```python
from build123d import *

# Parameters (mm, degrees)
SKETCH_R     = 11.1125
SKETCH003_R  = 11.1125
PAD_DEPTH    = 137
SKETCH004_W  = 152.4
SKETCH004_H  = 270.212156
PAD001_DEPTH = 0.508


with BuildPart() as part:
    # AdditivePipe: sweep along a path in Sketch001
    with BuildLine(Plane.YZ) as additivepipe_path:
        Line((0, 0), (279.4, 0))
        ThreePointArc((279.4, 0), (297.360512, -7.439488), (304.8, -25.4))
        Line((304.8, -25.4), (304.8, -254))
        ThreePointArc((304.8, -254), (297.360512, -271.960512), (279.4, -279.4))
        Line((279.4, -279.4), (184.15, -279.4))
        Line((184.15, -279.4), (184.15, -406.4))
        ThreePointArc((184.15, -406.4), (176.710512, -424.360512), (158.75, -431.8))
        Line((158.75, -431.8), (0, -431.8))
    # Sketch → AdditivePipe (sweep)
    with BuildSketch(Plane.XZ):
        Circle(SKETCH_R)
    sweep(path=additivepipe_path.line, transition=Transition.RIGHT)

    # Sketch003 (on DatumPlane) → Pad (new body)
    with BuildSketch(Plane(origin=(0, 69.85, -279.4), x_dir=(-1, 0, 0), z_dir=(0, 1, 0))):
        Circle(SKETCH003_R)
    extrude(amount=PAD_DEPTH)

    # Sketch004 → Pad001 (join, symmetric)
    with BuildSketch(Plane.YZ):
        with Locations((146.05, -138.737672)):
            Rectangle(SKETCH004_W, SKETCH004_H)
    extrude(amount=PAD001_DEPTH, both=True)


solid = part.part
```
CAD build for the part. Positions are in the model's coordinates, mm. A direction names the side the tool comes from. Give positions to 0.01 mm unless a question says otherwise; leave off trailing zeros. Put each result on its own line as item: value.
Q1. Tool access for faces 3 (the face through (-0.508, 145, -138)), 4 (the face through (-11.1, 183.66, -343.79)), 5 (the face through (0, 69.85, -233)), 6 (the face through (0.508, 145, -138)): list every direction of +Z, -Z, +X, -X, +Y, -Y with a clear straight run to the whole face (end or side of a thin tool).
Filled in:
face 3: -X, -Y
face 4: none
face 5: +X, -X, -Y
face 6: +X, -Y
Q2. Flat gauge pins, fed straight in: pin 1 (3 mm diameter, centred on x = -2, y = 67.5, fed in from +Z); pin 2 (4 mm diameter, centred on x = 1, z = -113, fed in from -Y); pin 3 (2 mm diameter, centred on y = 127.5, z = -71, fed in from -X). Where does each tip first touch, or does it go through?
Filled in:
pin 1: stops at z = 11.1
pin 2: stops at y = 69.85
pin 3: stops at x = -0.51
Q3. Mould opens along Z. For faces 1 (the face through (0, 0, -432)), 2 (the face through (10.6, 141.66, -3.34)) say: pulls with the +Z half, pulls with the -Z half, needs draft (parallel to the pull), parting line crosses it, or undercut.
Filled in:
face 1: needs draft
face 2: undercut
Q4. Probe line 1 along Z through (x, y) = (1, 74); line 2 along Y through (x, z) = (-0.25, -82); line 3 along Z through (x, y) = (9.75, 89). List the from-to ranges inside material, lowest first.
Filled in:
line 1: z = -442.87 to -420.73, -290.47 to -268.33, -11.07 to 11.07
line 2: y = 69.85 to 222.25, 293.69 to 315.91
line 3: z = -437.13 to -426.47, -284.73 to -274.07, -5.33 to 5.33
